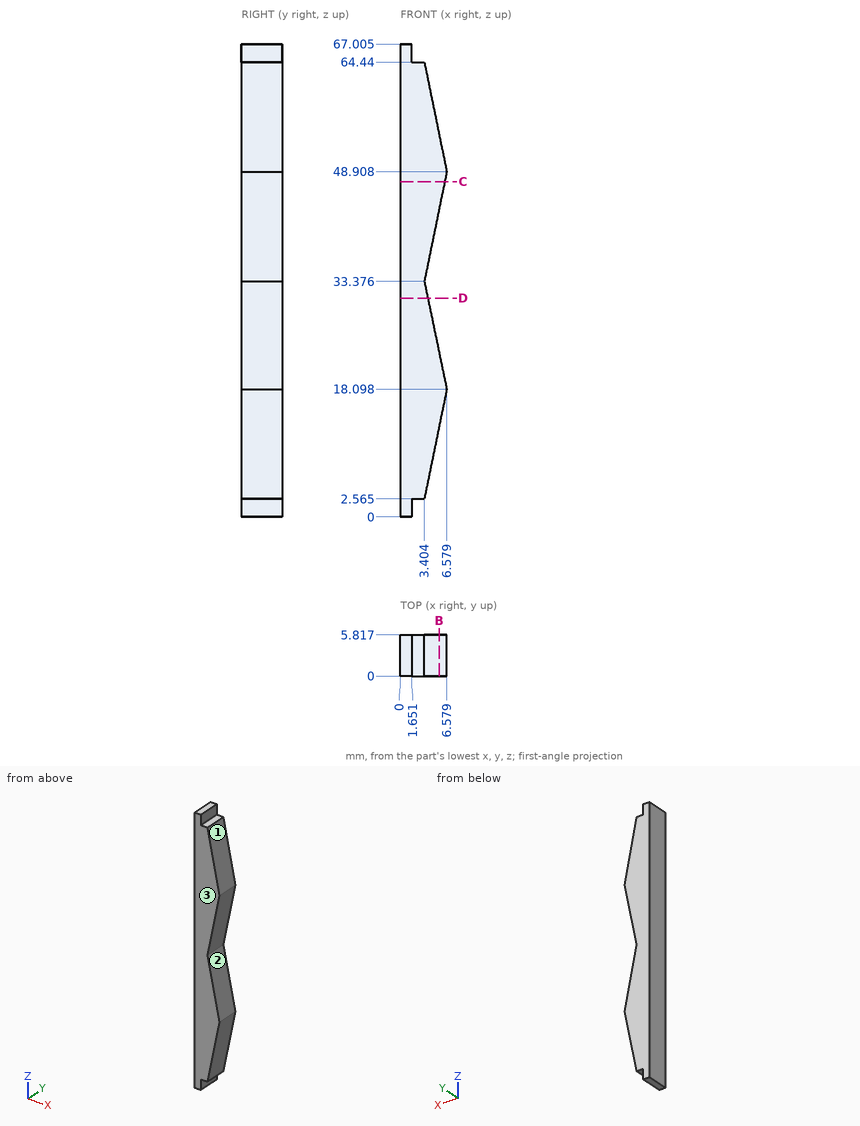
Design review of the part shown in the three views and the two pictorial views. Dimensions are in mm from the part's minimum x, y and z. Round coordinates to 2 decimals unless told otherwise and drop trailing zeros. Loops run counter-clockwise (first coordinate to the right, second up) from the corner with the lowest first, then second, coordinate; pieces in that order, holes last. Notation, with made-up numbers: M 47.5,79.5 L 63.5,79.5 A10 cw 63.5,90.5 Z; hole C 51.5,-37.75 d11. An arc over 180 degrees is marked long. Answer as a JSON object with one key per item and string values.
Item 1: We need section C-C, the plane z = 47.5. State the section outline as (x, y) points.
Check sheet entries:
{"outline": "M 0,0 L 6.29,0 L 6.29,5.82 L 0,5.82 Z"}
Item 2: The part is to be moulded in two halves that separate along Z. For the marked faces 1, 2 and 3, say which applies: +Z half, -Z half, draft (parallel to the pull), parting line (faces both ways), or undercut.
Check sheet entries:
{"face 1": "+Z half", "face 2": "undercut", "face 3": "draft"}
Item 3: Clearance check with flat-ended pins moving along their axes: P1, Ø3, axis at y = 3.5, z = 2, coming from the +X side (1 decimal); P2, Ø2, axis at y = 2.5, z = 65.5, coming from the +X side. State where each tip first meets the part, or that it passes through.
Check sheet entries:
{"P1": "x = 3.6", "P2": "x = 1.65"}
Item 4: We need section B-B, the plane x = 5.5. State the section outline as (y, z) points (1 decimal), and give its area (3 significant figures).
Check sheet entries:
{"outline": "M 0,12.8 L 5.8,12.8 L 5.8,23.3 L 0,23.3 Z; M 0,43.6 L 5.8,43.6 L 5.8,54.2 L 0,54.2 Z", "area": "122 mm2"}
Item 5: We need section D-D, the plane z = 31. State the section outline as (x, y) points.
Check sheet entries:
{"outline": "M 0,0 L 3.9,0 L 3.9,5.82 L 0,5.82 Z"}
Item 6: For line 1 along Z through (x, y) = (2.75, 4.2) (1 decimal); line 2 along X through (y, z) = (2.3, 41.5) (1 decimal); line 3 along X through (y, z) = (4.65, 5.5), list the stretches that pass through material, from the lowest coordinate up.
Check sheet entries:
{"line 1": "2.6 to 64.4", "line 2": "0 to 5.1", "line 3": "0 to 4"}
